```python
from build123d import *

# Parameters (mm, degrees)
BOSS_EXTRUDE1_DEPTH      = 200
BOSS_EXTRUDE1_DEPTH_BACK = 1600
SKETCH1_W                = 762
SKETCH1_H                = 762
CAVITY1_START            = -1500
CAVITY1_OUTLINE_R        = 304.8
CAVITY1_DEPTH            = 1600


# Read off the part's stored shape, not the designer's step: Cavity1
with BuildPart() as part:
    # Sketch1 → Boss-Extrude1 (new, two sides: drawn at the far end of the back side and taken through both)
    with BuildSketch(Plane(origin=(0, 0, 0), x_dir=(1, 0, 0), z_dir=(0, 1, 0)).offset(-BOSS_EXTRUDE1_DEPTH_BACK)):
        Rectangle(SKETCH1_W, SKETCH1_H)
    extrude(amount=BOSS_EXTRUDE1_DEPTH + BOSS_EXTRUDE1_DEPTH_BACK)

    # Cavity1 outline → Cavity1 (cut)
    with BuildSketch(Plane(origin=(0, 0, 0), x_dir=(1, 0, 0), z_dir=(0, 1, 0)).offset(CAVITY1_START)):
        Circle(CAVITY1_OUTLINE_R)
    extrude(amount=CAVITY1_DEPTH, mode=Mode.SUBTRACT)


solid = part.part
```
Geometry: final body of the model. Coordinates: model frame, mm. A direction names the side the tool comes from. Coordinates: 2 decimals unless noted, no trailing zeros. Write each loop counter-clockwise with the first axis right and the second up, starting at its lowest first coordinate (ties: lowest second). Pieces come first, ordered by that corner, then holes. Notation, with made-up numbers: M -35.75,75.5 L -0.75,75.5 A8 ccw -0.75,89.5 Z; hole C 1,-1 d10. An arc over 180 degrees is marked long. Answer as CSV lines item,"result". Start each with the question number.
Q1. Mould query, pull axis Y, two halves, no side actions, for faces 1 (the flat face through (-4, -1500, -4)), 2 (the flat face through (-5, -713, 381)), 3 (the flat face through (-5, -1600, -5)), 4 (the flat face through (-5, 200, -5)). Classes: released by +Y, released by -Y, zero draft, split by the parting line, or undercut.
Q2. Cut plane B-B on y = -253. Return the cut outline in (x, z), then the cut area to 3 significant figures.
Q3. Reachability of faces 5 (the flat face through (381, -713, 5)), 6 (the cylindrical face through (-241.879, -711.2, 185.466)) from +Z, -Z, +X, -X, +Y, -Y: full face, straight path, thin tool, end or side. Return the list, or none.
Q4. Cut plane A-A on x = 0. Return the cut outline in (y, z).
Q5. Cut plane C-C on z = 0. Return the cut outline in (x, y).
Q6. Line query: line 1 (Z direction, x = 0, y = -1040); line 2 (Y direction, x = 65, z = 83). Output: solid intervals per line, ascending. Write a range as from..to.
Findings below:
1,face 1,"undercut"
1,face 2,"zero draft"
1,face 3,"released by -Y"
1,face 4,"released by +Y"
2,outline,"M -381,-381 L 381,-381 L 381,381 L -381,381 Z; hole C 0,0 d609.6"
2,area,"289,000 mm2"
3,face 5,"+Z, -Z, +X, +Y, -Y"
3,face 6,"none"
4,outline,"M -1600,-381 L 200,-381 L 200,381 L -1600,381 Z; hole M -1500,-304.8 L 100,-304.8 L 100,304.8 L -1500,304.8 Z"
5,outline,"M -381,-1600 L 381,-1600 L 381,200 L -381,200 Z; hole M -304.8,-1500 L 304.8,-1500 L 304.8,100 L -304.8,100 Z"
6,line 1,"z = -381..-304.8, 304.8..381"
6,line 2,"y = -1600..-1500, 100..200"
